Input: dimensioned drawing with shaded views. Units: mm. Origin: part minimum x, y, z. Give positions to 0.01 mm unless a question says otherwise; leave off trailing zeros. Loops run counter-clockwise (first coordinate to the right, second up) from the corner with the lowest first, then second, coordinate; pieces in that order, holes last.
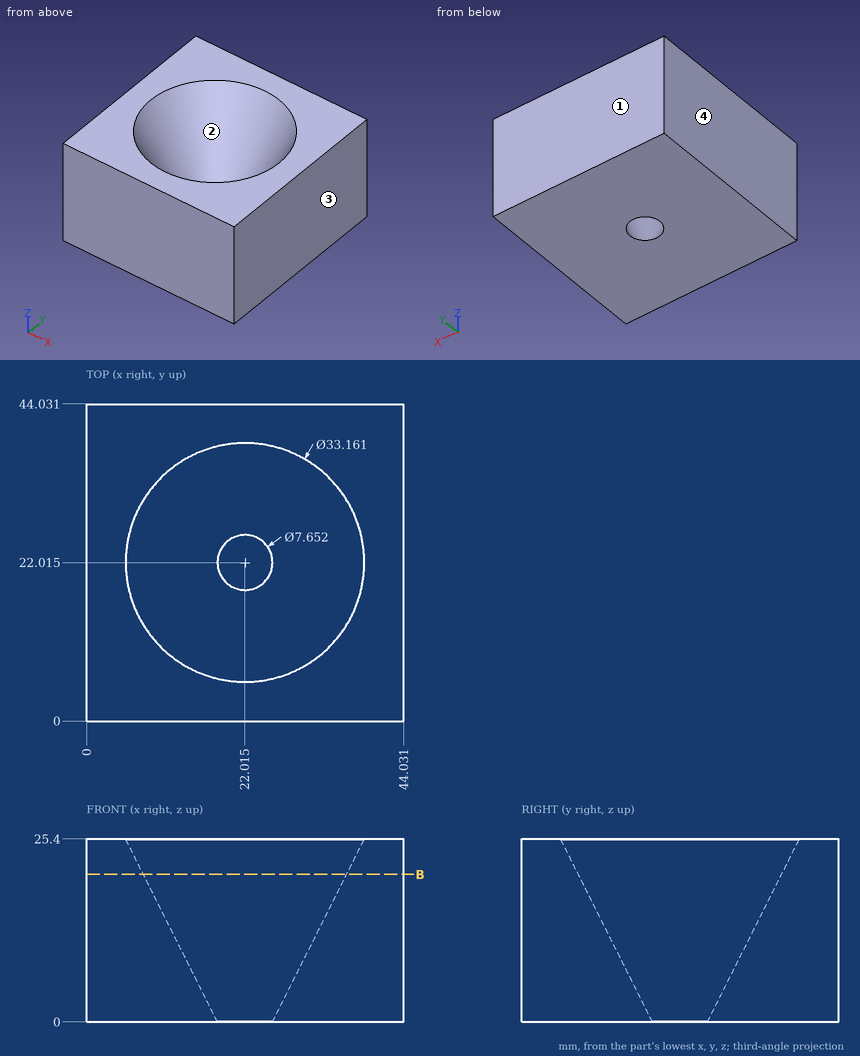
Item 1: Pin query (flat end, axial travel): pin 1 (8 mm diameter, centred on x = 33.5, z = 4.5, fed in from -Y). Return the tip coordinate at first contact, or that it passes through.
Values follow:
pin 1: stops at y = 0
Item 2: Draft query along X for the marked faces 1, 2, 3 and 4. Return one class per face: +X half, -X half, draft (parallel to the pull), parting line (faces both ways), or undercut.
Values follow:
face 1: draft
face 2: undercut
face 3: +X half
face 4: -X half
Item 3: Ray query, probe 1 along Y at (x, z) = (18.5, 17) (1 decimal); probe 2 along X at (y, z) = (25, 6.75) (1 decimal); probe 3 along Y at (x, z) = (22.5, 10.75) (1 decimal). Return the intervals inside material, ascending.
Values follow:
probe 1: y = 0 to 10.2, 33.9 to 44
probe 2: x = 0 to 15.4, 28.6 to 44
probe 3: y = 0 to 12.8, 31.2 to 44
Item 4: Section query B-B on z = 20.5. Return loops of the section in (x, y) (1 decimal).
Values follow:
outline: (0, 0) - (44, 0) - (44, 44) - (0, 44) - close; hole circle Ø28.2 at (22, 22)
